Verification items for the finished model (mm, model axes). Coordinates: 2 decimals unless noted, no trailing zeros. Write each loop counter-clockwise with the first axis right and the second up, starting at its lowest first coordinate (ties: lowest second). Pieces come first, ordered by that corner, then holes. Notation, with made-up numbers: (53, 43.5) -> (90, 43.5) arc R15 cw to (90, 69.5) -> close; hole circle Ø3 at (71, 1.5). An arc over 180 degrees is marked (long way). Use CSV: the item, a comma, the result in double quotes.
```python
from build123d import *

# Parameters (mm, degrees)
F0_R     = 9.7
F0_R_2   = 10.925
F1_DEPTH = 5


with BuildPart() as f1:
    # F0 (on Front) → F1 (new body)
    with BuildSketch(Plane.XZ):
        with BuildLine():
            ThreePointArc((8.31589, -12.516171), (15.015347, -0.00212), (8.282537, 12.494018))
            ThreePointArc((8.282537, 12.494018), (9.996409, 14.172211), (11.805892, 15.746843))
            ThreePointArc((11.805892, 15.746843), (23.94425, 22.617165), (37.687, 25))
            ThreePointArc((37.687, 25), (20.514782, 36.711637), (-0.009208, 39.999997))
            ThreePointArc((-0.009208, 39.999997), (-14.366945, 29.311716), (-8.267176, 12.483858))
            ThreePointArc((-8.267176, 12.483858), (-14.984626, -0.002104), (-8.300529, -12.505953))
            ThreePointArc((-8.300529, -12.505953), (-10.18297, -13.986049), (-11.805892, -15.746843))
            ThreePointArc((-11.805892, -15.746843), (-23.94425, -22.617165), (-37.687, -25))
            ThreePointArc((-37.687, -25), (-20.514782, -36.711637), (0.009208, -39.999997))
            ThreePointArc((0.009208, -39.999997), (14.358516, -29.339702), (8.31589, -12.516171))
        make_face()
        with Locations((0, -25)):
            Circle(F0_R, mode=Mode.SUBTRACT)
        Circle(F0_R_2, mode=Mode.SUBTRACT)
        with Locations((0, 25)):
            Circle(F0_R, mode=Mode.SUBTRACT)
    extrude(amount=F1_DEPTH)


solid = f1.part
```
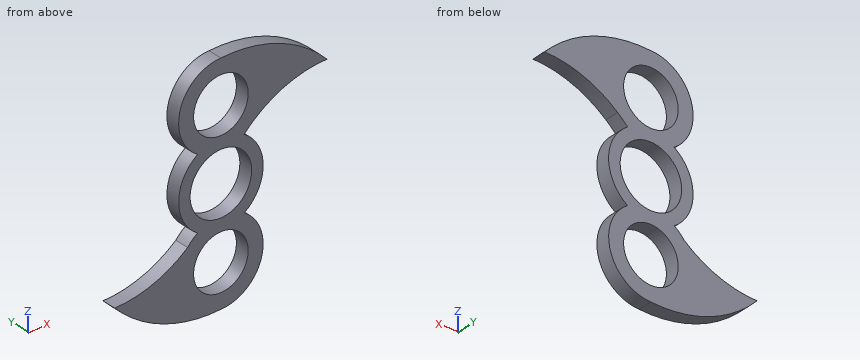
1) Cross-section at B-B (z = 28). Record the boundary of the cut face in (x, y).
Return value:
outline,"(-14.7, -5) -> (-9.22, -5) -> (-9.22, 0) -> (-14.7, 0) -> close; (9.22, -5) -> (34.61, -5) -> (34.61, 0) -> (9.22, 0) -> close"
2) Scan lines: L1, parallel to Z at x = 0, y = -2.7 (3 decimals); L2, parallel to Z at x = -1.5, y = -3.2; L3, parallel to X at y = -2.05, z = -7. Record each from-to range of solid material in increasing order.
Return value:
L1,"-40.001 to -34.7, -15.3 to -10.925, 10.925 to 15.3, 34.7 to 40.001"
L2,"-40.07 to -34.58, -15.42 to -10.82, 10.82 to 15.42, 34.58 to 39.92"
L3,"-13.26 to -8.39, 8.39 to 13.29"
3) Cross-section at D-D (x = -13). Record the boundary of the cut face in (y, z), plus the area to 3 significant figures.
Return value:
outline,"(-5, -39) -> (0, -39) -> (0, -16.69) -> (-5, -16.69) -> close; (-5, -7.48) -> (0, -7.48) -> (0, 7.43) -> (-5, 7.43) -> close; (-5, 17.52) -> (0, 17.52) -> (0, 32.48) -> (-5, 32.48) -> close"
area,"261 mm2"
4) Gauge pin test, flat end, axial feed: pin 1 (2 mm diameter, centred on y = -3.5, z = -24, fed in from +X). Record the tip position at first contact, or that the pin passes through.
Return value:
pin 1,"x = 15"
5) Cross-section at A-A (x = 3). Record the boundary of the cut face in (y, z).
Return value:
outline,"(-5, -39.7) -> (0, -39.7) -> (0, -34.22) -> (-5, -34.22) -> close; (-5, -15.78) -> (0, -15.78) -> (0, -10.51) -> (-5, -10.51) -> close; (-5, 10.51) -> (0, 10.51) -> (0, 15.78) -> (-5, 15.78) -> close; (-5, 34.22) -> (0, 34.22) -> (0, 40.09) -> (-5, 40.09) -> close"
6) Cross-section at C-C (y = -2.1). Record the boundary of the cut face in (x, z) (3 decimals), plus the area to 3 significant figures.
Return value:
outline,"(-37.687, -25) arc R47.658 ccw to (0.009, -40) arc R15 ccw to (8.316, -12.516) arc R15 ccw to (8.283, 12.494) arc R40.821 cw to (11.806, 15.747) arc R40.821 cw to (37.687, 25) arc R47.658 ccw to (-0.009, 40) arc R15 ccw to (-8.267, 12.484) arc R15 ccw to (-8.301, -12.506) arc R15 ccw to (-11.806, -15.747) arc R40.821 cw to start; hole circle Ø21.85 at (0, 0); hole circle Ø19.4 at (0, -25); hole circle Ø19.4 at (0, 25)"
area,"1,610 mm2"
